Can you work these out from the drawing? Everything is in mm from the part's minimum corner. Give positions to 0.01 mm unless a question says otherwise; leave off trailing zeros. Write each loop counter-clockwise with the first axis right and the second up, starting at its lowest first coordinate (ties: lowest second). Pieces come first, ordered by that corner, then holes. Notation, with made-up numbers: (47, 19.5) -> (105, 19.5) arc R18 cw to (105, 37.5) -> close; hole circle Ø6 at (10.5, -7). An arc over 180 degrees is marked (long way). Use one line per item in the form item = value.
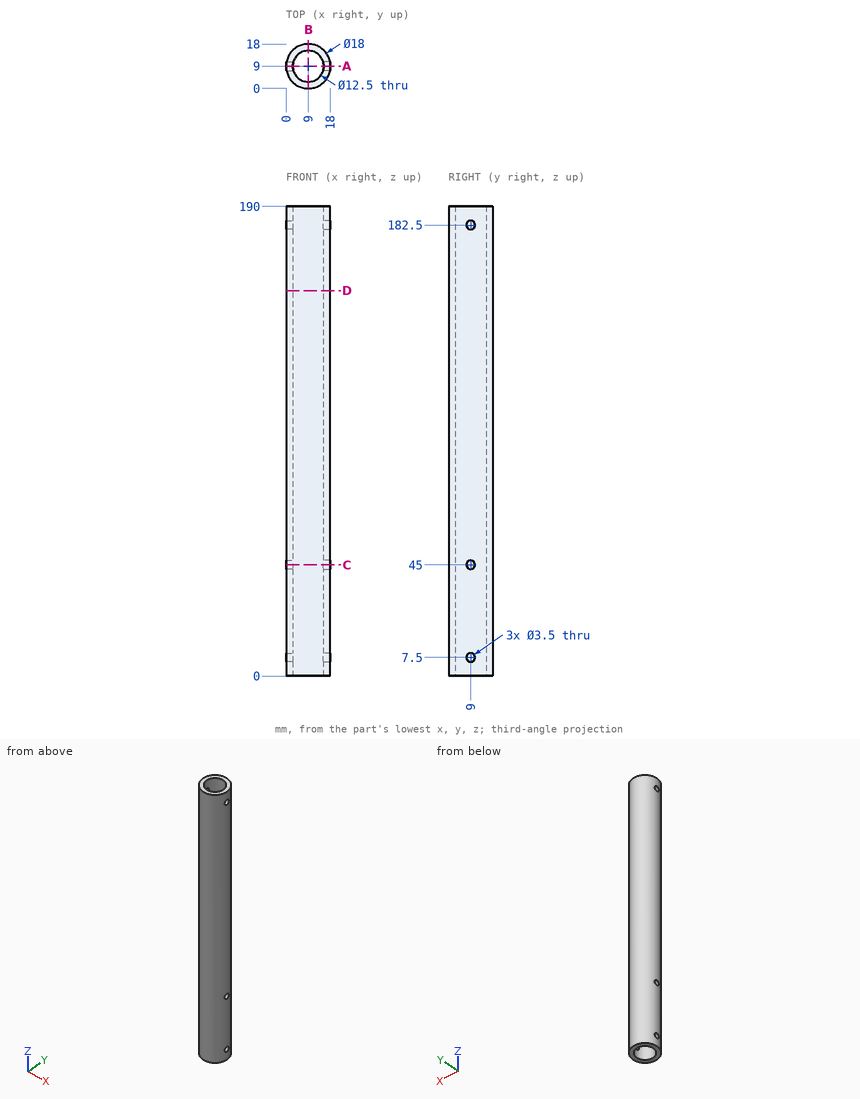
Q1. I want a section at B-B, the plane x = 9. Write out the boundary of the cut face in (y, z).
Result set:
outline = (0, 0) -> (2.75, 0) -> (2.75, 190) -> (0, 190) -> close; (15.25, 0) -> (18, 0) -> (18, 190) -> (15.25, 190) -> close
Q2. Will these pins go through, and if not, where does the flat tip stop? pin 1 Ø3 at (y, z) = (9, 7.5) entering from +X; pin 2 Ø1 at (y, z) = (14, 25) entering from +X; pin 3 Ø1 at (y, z) = (10.5, 128.5) entering from -X.
Result set:
pin_1 = through
pin_2 = 16.79
pin_3 = 0.06
Q3. I want a section at A-A, the plane y = 9. Count the separate pieces of the cut face and the enclosed holes in it, and give its area (3 significant figures).
Result set:
separate_pieces = 8
enclosed_holes = 0
area = 987 mm2
Q4. If I drill on line 1 along Y through (x, z) = (8.75, 39.5) (3 decimals); line 2 along Y through (x, z) = (2.5, 29.5); line 3 along X through (y, z) = (14, 111.5), over which ranges is the centre line in solid material (lowest first)? Write a range as from..to.
Result set:
line_1 = 0.003..2.755, 15.245..17.997
line_2 = 2.78..15.22
line_3 = 1.52..5.25, 12.75..16.48
Q5. I want a section at C-C, the plane z = 45. Write out the boundary of the cut face in (x, y).
Result set:
outline = (0.17, 7.25) arc R9 ccw to (17.83, 7.25) -> (15, 7.25) arc R6.25 cw to (3, 7.25) -> close; (0.17, 10.75) -> (3, 10.75) arc R6.25 cw to (15, 10.75) -> (17.83, 10.75) arc R9 ccw to start
Q6. I want a section at D-D, the plane z = 156. Write out the boundary of the cut face in (x, y).
Result set:
outline = circle Ø18 at (9, 9); hole circle Ø12.5 at (9, 9)
